Check sheet for the modelled part. Datum: model origin and axes. Units: mm. Coordinates: 2 decimals unless noted, no trailing zeros. Loops run counter-clockwise (first coordinate to the right, second up) from the corner with the lowest first, then second, coordinate; pieces in that order, holes last.
```python
from build123d import *

# Parameters (mm, degrees)
BLANKSKE_W          = 203.2
BLANKSKE_H          = 28.575
BLANK_DEPTH         = 11.811
TOOTHCUTILL_DEPTH   = 12.811
TOOTHCUTSIM_DEPTH   = 12.811
TEETHCUTS_COUNT     = 22
TEETHCUTS_PITCH     = 9.974556664
SKETCH1_W           = 44.45
SKETCH1_H           = 38.1
BOSS_EXTRUDE1_DEPTH = 11.811
SKETCH2_R           = 3.175
CUT_EXTRUDE1_DEPTH  = 12.811


with BuildPart() as part:
    # BlankSke → Blank (new body)
    with BuildSketch(Plane.XY):
        with Locations((101.6, 14.2875)):
            Rectangle(BLANKSKE_W, BLANKSKE_H)
    extrude(amount=-BLANK_DEPTH)

    # TooCutSkeIll → ToothCutIll (cut, through all)
    with BuildSketch(Plane.XY):
        with BuildLine():
            Line((-3.961730054, 28.491436558), (-1.582427729, 21.954357146))
            ThreePointArc((-1.582427729, 21.954357146), (-1.29135804, 21.575027742), (-0.835353302, 21.43125))
            Line((-0.835353302, 21.43125), (0.835353302, 21.43125))
            ThreePointArc((0.835353302, 21.43125), (1.29135804, 21.575027742), (1.582427729, 21.954357146))
            Line((1.582427729, 21.954357146), (3.961730054, 28.491436558))
            ThreePointArc((3.961730054, 28.491436558), (4.00822681, 28.55203231), (4.081071017, 28.575))
            Line((4.081071017, 28.575), (4.081071017, 28.6004))
            Line((4.081071017, 28.6004), (-4.081071017, 28.6004))
            Line((-4.081071017, 28.6004), (-4.081071017, 28.575))
            ThreePointArc((-4.081071017, 28.575), (-4.00822681, 28.55203231), (-3.961730054, 28.491436558))
        make_face()
    toothcutill = extrude(amount=-TOOTHCUTILL_DEPTH, mode=Mode.SUBTRACT)

    # TooCutSkeSim → ToothCutSim (cut, through all)
    with BuildSketch(Plane.XY):
        Polygon((1.392032299, 21.43125), (-1.392032299, 21.43125), (-4.001389504, 28.6004), (4.001389504, 28.6004), align=None)
    toothcutsim = extrude(amount=-TOOTHCUTSIM_DEPTH, mode=Mode.SUBTRACT)

    # TeethCuts: ToothCutIll, ToothCutSim ×22
    with Locations(*[(i * TEETHCUTS_PITCH, 0, 0) for i in range(1, TEETHCUTS_COUNT)]):
        add(toothcutill, mode=Mode.SUBTRACT)
        add(toothcutsim, mode=Mode.SUBTRACT)

    # Sketch1 → Boss-Extrude1 (add)
    with BuildSketch(Plane.XY):
        with Locations((22.225, 19.05)):
            Rectangle(SKETCH1_W, SKETCH1_H)
    extrude(amount=-BOSS_EXTRUDE1_DEPTH)

    # Sketch2 → Cut-Extrude1 (cut, through all)
    with BuildSketch(Plane.XY):
        with Locations((9.525, 28.575)):
            Circle(SKETCH2_R)
        with Locations((9.525, 9.525)):
            Circle(SKETCH2_R)
    extrude(amount=-CUT_EXTRUDE1_DEPTH, mode=Mode.SUBTRACT)


solid = part.part
```
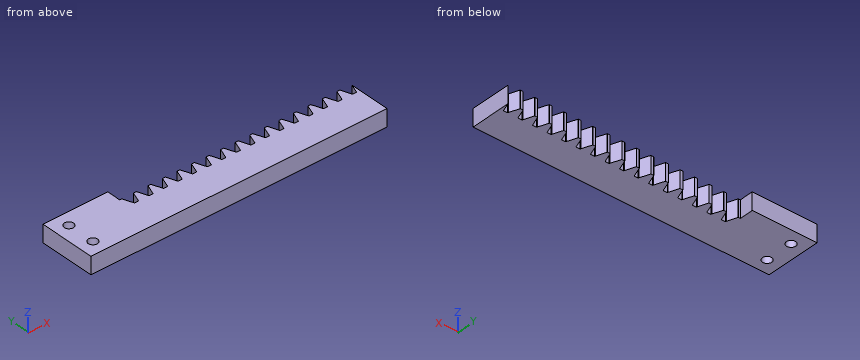
1) Scan lines: line 1 (Y direction, x = 11, z = -3.25); line 2 (X direction, y = 9, z = -2.25); line 3 (X direction, y = 31.5, z = -6). Record each from-to range of solid material in increasing order.
Answer sheet:
line 1: y = 0 to 6.71, 12.34 to 25.76, 31.39 to 38.1
line 2: x = 0 to 6.39, 12.66 to 203.2
line 3: x = 0 to 8.29, 10.76 to 44.45
2) Depth check by flat-ended pin: pin 1 (1.4 mm diameter, centred on x = 199, z = -8.5, fed in from +Y); pin 2 (2 mm diameter, centred on x = 104.5, z = -5, fed in from +Y) (3 decimals); pin 3 (5 mm diameter, centred on y = 32, z = -6, fed in from +X). Enter the tip coordinate at first touch or a pass-through.
Answer sheet:
pin 1: stops at y = 21.43
pin 2: stops at y = 28.575
pin 3: stops at x = 44.45
3) Section check B-B on z = -2.75. Give the number of separate pieces and of enclosed holes in the cut face, plus the area to 3 significant figures.
Answer sheet:
separate pieces: 1
enclosed holes: 2
area: 5,550 mm2
4) Section check A-A on y = 35.5. Enter the section's corners in (x, z).
Answer sheet:
outline: (0, -11.81) - (44.45, -11.81) - (44.45, 0) - (0, 0) - close
